Geometry check sheet. Reference: the model listing, model coordinates, mm. Give positions to 0.01 mm unless a question says otherwise; leave off trailing zeros. Order: outer loops, then holes, each group sorted by start corner. A loop starts at its lowest first (then second) coordinate and runs counter-clockwise, first axis right, second up. Notation, with made-up numbers: M 80,26 L 128,26 A33 cw 128,63 Z; hole C 9,64 d1. An arc over 180 degrees is marked long. Put each result on its own line as item: value. Start each with the question number.
Q1. Section check D-D on y = 0.05. Record the cut outline in (x, z), then the cut area to 3 significant figures.
Q2. Section check C-C on z = 12.1. Record the cut outline in (x, y), then the cut area to 3 significant figures.
Q3. Material ranges on L1, parallel to X at y = 0.05, z = 12.15; L2, parallel to Z at x = -32, y = 0.05; L3, parallel to Z at x = -34, y = 0.05, recorded low to high.
Q4. Section check B-B on z = 13.1. Record the cut outline in (x, y), then the cut area to 3 significant figures.
Q5. Section check A-A on z = 13.95. Record the cut outline in (x, y), then the cut area to 3 significant figures.
```python
from build123d import *

# Parameters (mm, degrees)
SKETCH1_R           = 1.5875
BOSS_EXTRUDE1_DEPTH = 1.65
SKETCH2_R           = 0.4
CUT_EXTRUDE1_DEPTH  = 1.65
SKETCH3_R           = 0.4
CUT_EXTRUDE2_DEPTH  = 1.65
LPATTERN1_COUNT     = 15
LPATTERN1_PITCH     = 2.54
SKETCH4_R           = 0.4
CUT_EXTRUDE3_DEPTH  = 1.65
LPATTERN2_COUNT     = 10
LPATTERN2_PITCH     = 2.54
EXTRUDE_1_DEPTH     = 0.1
SKETCH_2_W          = 71.696119323
SKETCH_2_H          = 83.90888514
CUT_EXTRUDE_1_DEPTH = 87.897033896


with BuildPart() as part:
    # Sketch1 → Boss-Extrude1 (new body)
    with BuildSketch(Plane(origin=(0, 0, 0), x_dir=(1, 0, 0), z_dir=(0, 1, 0))):
        Polygon((0, 0), (-53.34, 0), (-53.34, 66.04), (-40.386, 66.04), (-37.846, 68.58), (-5.08, 68.58), (-2.54, 66.04), (0, 66.04), align=None)
        with Locations(Location((-7.62, 66.04, 0), (0, 0, 270))):
            Circle(SKETCH1_R, mode=Mode.SUBTRACT)
        with Locations(Location((-35.56, 66.04, 0), (0, 0, 270))):
            Circle(SKETCH1_R, mode=Mode.SUBTRACT)
        with Locations(Location((-2.54, 13.97, 0), (0, 0, 270))):
            Circle(SKETCH1_R, mode=Mode.SUBTRACT)
        with Locations(Location((-50.8, 15.24, 0), (0, 0, 270))):
            Circle(SKETCH1_R, mode=Mode.SUBTRACT)
    extrude(amount=-BOSS_EXTRUDE1_DEPTH)

    # Sketch2 → Cut-Extrude1 (cut)
    with BuildSketch(Plane(origin=(0, 0, 0), x_dir=(1, 0, 0), z_dir=(0, 1, 0))):
        with Locations(Location((-2.54, 27.94, 0), (0, 0, 270))):
            Circle(SKETCH2_R)
    cut_extrude1 = extrude(amount=-CUT_EXTRUDE1_DEPTH, mode=Mode.SUBTRACT)

    # Sketch3 → Cut-Extrude2 (cut)
    with BuildSketch(Plane(origin=(0, 0, 0), x_dir=(1, 0, 0), z_dir=(0, 1, 0))):
        with Locations(Location((-50.8, 18.796, 0), (0, 0, 270))):
            Circle(SKETCH3_R)
    cut_extrude2 = extrude(amount=-CUT_EXTRUDE2_DEPTH, mode=Mode.SUBTRACT)

    # LPattern1: Cut-Extrude1 ×15, 1 skipped
    with Locations(*[(0, 0, -i * LPATTERN1_PITCH) for i in range(1, LPATTERN1_COUNT) if i not in (8,)]):
        add(cut_extrude1, mode=Mode.SUBTRACT)

    # Sketch4 → Cut-Extrude3 (cut)
    with BuildSketch(Plane(origin=(0, 0, 0), x_dir=(1, 0, 0), z_dir=(0, 1, 0))):
        with Locations(Location((-50.8, 45.72, 0), (0, 0, 270))):
            Circle(SKETCH4_R)
    extrude(amount=-CUT_EXTRUDE3_DEPTH, mode=Mode.SUBTRACT)

    # LPattern2: Cut-Extrude2 ×10
    with Locations(*[(0, 0, -i * LPATTERN2_PITCH) for i in range(1, LPATTERN2_COUNT)]):
        add(cut_extrude2, mode=Mode.SUBTRACT)

    # 草图2 → 切除-拉伸1 (cut, through all)
    with BuildSketch(Plane(origin=(0, 0, 0), x_dir=(1, 0, 0), z_dir=(0, 1, 0))):
        with Locations((-23.858381216, 34.717351285)):
            Rectangle(SKETCH_2_W, SKETCH_2_H)
    extrude(amount=-CUT_EXTRUDE_1_DEPTH, mode=Mode.SUBTRACT)


with BuildPart() as body_2:
    # 草图1 → 凸台-拉伸1 (new body)
    with BuildSketch(Plane(origin=(0, 0, 0), x_dir=(1, 0, 0), z_dir=(0, 1, 0))):
        Polygon((-37.34, -11.757389562), (-37.34, -16.957389562), (-34.54, -16.957389562), (-34.54, -13.357389562), (-32.74, -13.357389562), (-32.74, -16.957389562), (-29.84, -16.957389562), (-29.84, -13.357389562), (-28.04, -13.357389562), (-28.04, -16.957389562), (-22.94, -16.957389562), (-22.94, -10.957389562), (-23.74, -10.957389562), (-23.74, -16.357389562), (-25.24, -16.357389562), (-25.24, -10.957389562), (-25.84, -10.957389562), (-25.84, -16.357389562), (-27.34, -16.357389562), (-27.34, -12.757389562), (-30.44, -12.757389562), (-30.44, -16.357389562), (-32.14, -16.357389562), (-32.14, -12.757389562), (-35.14, -12.757389562), (-35.14, -16.357389562), (-36.74, -16.357389562), (-36.74, -11.757389562), align=None)
    extrude(amount=EXTRUDE_1_DEPTH)


solid = body_2.part
```
Results found:
1. outline: M -37.34,11.76 L -36.74,11.76 L -36.74,16.36 L -35.14,16.36 L -35.14,12.76 L -32.14,12.76 L -32.14,16.36 L -30.44,16.36 L -30.44,12.76 L -27.34,12.76 L -27.34,16.36 L -25.84,16.36 L -25.84,10.96 L -25.24,10.96 L -25.24,16.36 L -23.74,16.36 L -23.74,10.96 L -22.94,10.96 L -22.94,16.96 L -28.04,16.96 L -28.04,13.36 L -29.84,13.36 L -29.84,16.96 L -32.74,16.96 L -32.74,13.36 L -34.54,13.36 L -34.54,16.96 L -37.34,16.96 Z
1. area: 28.0 mm^2
2. outline: M -37.34,0 L -36.74,0 L -36.74,0.1 L -37.34,0.1 Z; M -25.84,0 L -25.24,0 L -25.24,0.1 L -25.84,0.1 Z; M -23.74,0 L -22.94,0 L -22.94,0.1 L -23.74,0.1 Z
2. area: 0.200 mm^2
3. L1: x = -37.34 to -36.74, -25.84 to -25.24, -23.74 to -22.94
3. L2: z = 16.36 to 16.96
3. L3: z = 12.76 to 13.36
4. outline: M -37.34,0 L -36.74,0 L -36.74,0.1 L -37.34,0.1 Z; M -35.14,0 L -32.14,0 L -32.14,0.1 L -35.14,0.1 Z; M -30.44,0 L -27.34,0 L -27.34,0.1 L -30.44,0.1 Z; M -25.84,0 L -25.24,0 L -25.24,0.1 L -25.84,0.1 Z; M -23.74,0 L -22.94,0 L -22.94,0.1 L -23.74,0.1 Z
4. area: 0.810 mm^2
5. outline: M -37.34,0 L -36.74,0 L -36.74,0.1 L -37.34,0.1 Z; M -35.14,0 L -34.54,0 L -34.54,0.1 L -35.14,0.1 Z; M -32.74,0 L -32.14,0 L -32.14,0.1 L -32.74,0.1 Z; M -30.44,0 L -29.84,0 L -29.84,0.1 L -30.44,0.1 Z; M -28.04,0 L -27.34,0 L -27.34,0.1 L -28.04,0.1 Z; M -25.84,0 L -25.24,0 L -25.24,0.1 L -25.84,0.1 Z; M -23.74,0 L -22.94,0 L -22.94,0.1 L -23.74,0.1 Z
5. area: 0.450 mm^2
